from build123d import *

# Parameters (mm, degrees)
F1_DEPTH = 63.5
F0_W     = 25.4
F0_H     = 19.05
F2_DEPTH = 25.4
F3_DEPTH = 7.9375
F5_R     = 6.35


with BuildPart() as f1:
    # F0 (on Front) → F1 (new body, symmetric)
    with BuildSketch(Plane.XZ):
        Polygon((22.225, 9.525), (-41.275, 9.525), (-41.275, -9.525), (41.275, -9.525), (41.275, 9.525), align=None)
    extrude(amount=F1_DEPTH, both=True)

    # F0 (on Front) → F2 (join, symmetric)
    with BuildSketch(Plane.XZ):
        with BuildLine():
            Line((22.225, 27.0002), (22.225, 9.525))
            Line((22.225, 9.525), (41.275, 9.525))
            Line((41.275, 9.525), (41.275, 27.0002))
            ThreePointArc((41.275, 27.0002), (45.9246798487, 38.2255201513), (57.15, 42.8752))
            Line((57.15, 42.8752), (58.465048489, 42.8752))
            Line((58.465048489, 42.8752), (58.465048489, 61.9252))
            Line((58.465048489, 61.9252), (57.15, 61.9252))
            add(Edge.make_bspline(
                [(56.1593998767, 61.9111486608), (56.4890557248, 61.9164037237), (56.8192573531, 61.9210875625), (57.15, 61.9252)],
                knots=[110.8592289818, 110.8592289818, 110.8592289818, 110.8592289818, 111.5045361635, 111.5045361635, 111.5045361635, 111.5045361635], degree=3))
            ThreePointArc((56.1593998767, 61.9111486608), (32.1065144768, 51.3431549941), (22.225, 27.0002))
        make_face()
        with Locations((71.165048489, 52.4002)):
            Rectangle(F0_W, F0_H)
        Polygon((83.865048489, 66.675), (83.865048489, 61.9252), (83.865048489, 42.8752), (83.865048489, 38.1), (109.265048489, 38.1), (109.265048489, 66.675), align=None)
    extrude(amount=F2_DEPTH, both=True)

    # F0 (on Front) → F3 (join, symmetric)
    with BuildSketch(Plane.XZ):
        with BuildLine():
            add(Edge.make_bspline(
                [(-41.275, 9.525), (-40.9981963046, 43.2471461139), (-0.4731530978, 61.0083658582), (56.1593998767, 61.9111486608)],
                knots=[0, 0, 0, 0, 110.8592289818, 110.8592289818, 110.8592289818, 110.8592289818], degree=3))
            Line((-41.275, 9.525), (22.225, 9.525))
            Line((22.225, 9.525), (22.225, 27.0002))
            ThreePointArc((22.225, 27.0002), (32.1065144768, 51.3431549941), (56.1593998767, 61.9111486608))
        make_face()
    extrude(amount=F3_DEPTH, both=True)

    # F0 (on Front) → F4 (revolve)
    with BuildSketch(Plane.XZ):
        Polygon((83.865048489, 66.675), (83.865048489, 61.9252), (83.865048489, 42.8752), (83.865048489, 38.1), (109.265048489, 38.1), (109.265048489, 66.675), align=None)
    revolve(axis=Axis((83.865048489, 0, 52.3875), (0, 0, 1)))

    # F5
    f5_edges = [f1.edges().sort_by_distance(p)[0] for p in [
        (-41.275, 63.5, 0),
        (-41.275, -63.5, 0),
        (41.275, -63.5, 0),
        (41.275, 63.5, 0),
    ]]
    fillet(f5_edges, radius=F5_R)


solid = f1.part
Part model, mm, in its own coordinate system. A direction names the side the tool comes from. Round coordinates to 2 decimals unless told otherwise and drop trailing zeros. Loops run counter-clockwise (first coordinate to the right, second up) from the corner with the lowest first, then second, coordinate; pieces in that order, holes last. Notation, with made-up numbers: (40.25, 87) - (63.25, 87) arc R12 ccw to (63.25, 104) - close; hole circle Ø1 at (14, -38). An arc over 180 degrees is marked (long way). Answer as a JSON object with one key per item and string values.
Item 1: Band-saw the part on A-A on y = 51. List the corners of the cut face in (x, z) (3 decimals).
Output:
{"outline": "(-41.275, -9.525) - (41.275, -9.525) - (41.275, 9.525) - (-41.275, 9.525) - close"}
Item 2: Pin check, flat tips, straight feed: pin 1 (8 mm diameter, centred on x = 66, y = 7.5, fed in from -Z); pin 2 (4 mm diameter, centred on x = -22.5, z = 38, fed in from -Y); pin 3 (12 mm diameter, centred on x = -18.5, z = 20, fed in from +Y). Stop position of each tip, or through.
Output:
{"pin 1": "z = 38.1", "pin 2": "y = -7.94", "pin 3": "y = 7.94"}
Item 3: Band-saw the part on B-B on x = 96.5. List the corners of the cut face in (y, z) (3 decimals), plus the area to 3 significant figures.
Output:
{"outline": "(-25.4, 38.1) - (25.4, 38.1) - (25.4, 66.675) - (-25.4, 66.675) - close", "area": "1,450 mm2"}
Item 4: Tool access for faces 1 (the face through (22.225, -17, 18)), 2 (the face through (58.6, -3.9, 42.875)), 3 (the face through (22.225, 17, 18)), 4 (the face through (58, 4, 61.925)), 5 (the face through (65, 25.4, 45)): list every direction of +Z, -Z, +X, -X, +Y, -Y with a clear straight run to the whole face (end or side of a thin tool).
Output:
{"face 1": "+Z, -X, -Y", "face 2": "-Z", "face 3": "+Z, -X, +Y", "face 4": "+Z, -X", "face 5": "+Z, +X, -X, +Y"}
Item 5: Wall check: L1, parallel to Z at x = -14, y = -13.5 (3 decimals); L2, parallel to Y at x = 30.5, z = 25; L3, parallel to Y at x = 14.5, z = 20. Give the ranges that are in metal, low to high.
Output:
{"L1": "-9.525 to 9.525", "L2": "-25.4 to 25.4", "L3": "-7.94 to 7.94"}
Item 6: Pull direction X, two halves, no side cores. Call faces 6 (the face through (1, 35, 9.525)), 7 (the face through (45.8, -0.4, 38.1)), 8 (the face through (-39.464, 61.59, -0.133)): pulls with the +X half, pulls with the -X half, needs draft (parallel to the pull), parting line crosses it, or undercut.
Output:
{"face 6": "needs draft", "face 7": "undercut", "face 8": "pulls with the -X half"}
